Here's the drawing with two shaded views (mm, measured from the low corner). I have some questions. A direction names the side the tool comes from. Coordinates: 2 decimals unless noted, no trailing zeros. Loops run counter-clockwise (first coordinate to the right, second up) from the corner with the lowest first, then second, coordinate; pieces in that order, holes last.
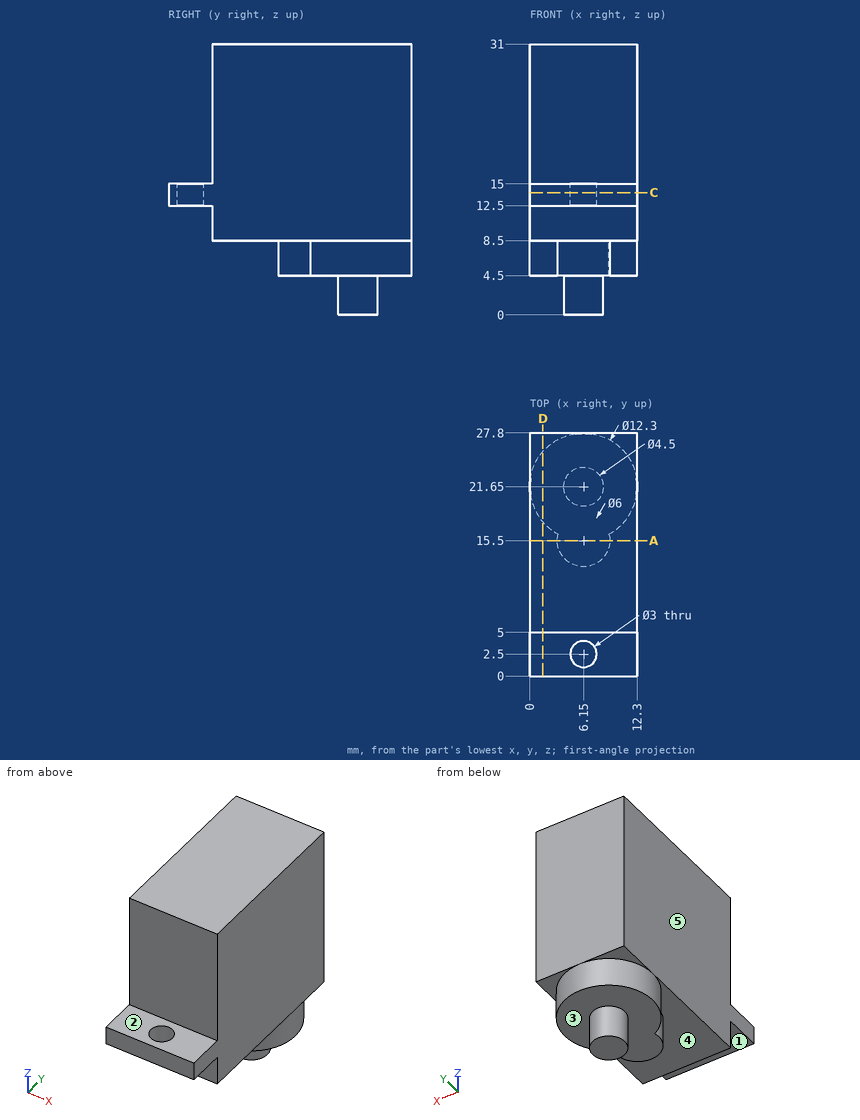
(1) I want a section at D-D on x = 1.5. Write out the boundary of the cut face in (y, z), then the cut area to 3 significant figures.
Check values:
outline: (0, 12.5) - (5, 12.5) - (5, 8.5) - (17.63, 8.5) - (17.63, 4.5) - (25.67, 4.5) - (25.67, 8.5) - (27.8, 8.5) - (27.8, 31) - (5, 31) - (5, 15) - (0, 15) - close
area: 558 mm2
(2) Which directions (+Z, -Z, +X, -X, +Y, -Y) give clear straight access to the entire face, cutting with the end or side of a thin tool? Please do the marked faces 1, 2, 3, 4 and 5.
Check values:
face 1: -Z, +X, -X, -Y
face 2: +Z, +X, -X, -Y
face 3: -Z
face 4: -Z, -Y
face 5: +Z, -Z, -X, +Y, -Y
(3) I want a section at C-C on z = 14. Write out the boundary of the cut face in (x, y).
Check values:
outline: (0, 0) - (12.3, 0) - (12.3, 27.8) - (0, 27.8) - close; hole circle Ø3 at (6.15, 2.5)
(4) I want a section at A-A on y = 15.5. Write out the boundary of the cut face in (x, z).
Check values:
outline: (0, 8.5) - (3.15, 8.5) - (3.15, 4.5) - (9.15, 4.5) - (9.15, 8.5) - (12.3, 8.5) - (12.3, 31) - (0, 31) - close
(5) If I drill on probe 1 along X at (y, z) = (2.5, 14.05); probe 2 along Y at (x, z) = (4.5, 20); probe 3 along Z at (x, y) = (4.75, 25.25), over which ranges is the centre line in solid material (lowest first)?
Check values:
probe 1: x = 0 to 4.65, 7.65 to 12.3
probe 2: y = 5 to 27.8
probe 3: z = 4.5 to 31
(6) I'm going to push flat-ended pins straight in: pin 1 (5.5 mm diameter, centred on x = 4, y = 2, fed in from -Z); pin 2 (4 mm diameter, centred on x = 6.15, y = 2.5, fed in from +Z); pin 3 (6 mm diameter, centred on x = 3.5, y = 16, fed in from -Z); pin 4 (6 mm diameter, centred on x = 5.5, y = 17.5, fed in from -Z). Where does each tip first touch, or does it pass through?
Check values:
pin 1: stops at z = 12.5
pin 2: stops at z = 15
pin 3: stops at z = 4.5
pin 4: stops at z = 0
